Read the model definition and answer for the solid it produces. Units are mm, in the model's axes. Face numbers are marked on the shaded views. Coordinates: 2 decimals unless noted, no trailing zeros. Order: outer loops, then holes, each group sorted by start corner. A loop starts at its lowest first (then second) coordinate and runs counter-clockwise, first axis right, second up. Notation, with made-up numbers: (-15.5, 33) -> (27.5, 33) arc R5 cw to (27.5, 39) -> close; hole circle Ø9 at (33.5, 53.25). An arc over 180 degrees is marked (long way). Answer in a Markdown table with one row per item.
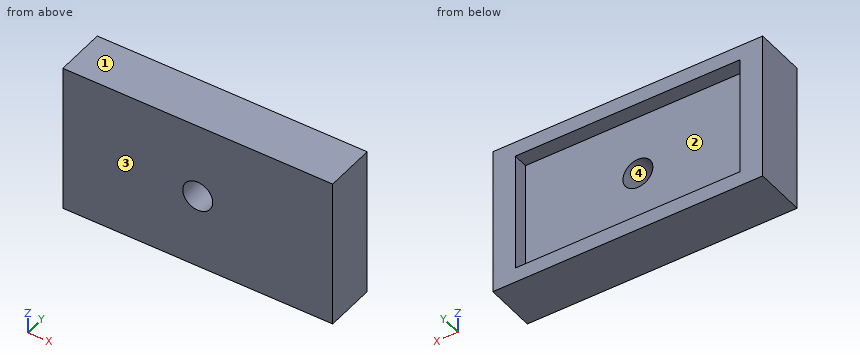
from build123d import *

# Parameters (mm, degrees)
SKETCH1_W           = 90
SKETCH1_H           = 50
BOSS_EXTRUDE1_DEPTH = 17
SKETCH2_W           = 75
SKETCH2_H           = 40
CUT_EXTRUDE1_DEPTH  = 5
SKETCH3_R           = 5
CUT_EXTRUDE2_DEPTH  = 13


with BuildPart() as part:
    # Sketch1 → Boss-Extrude1 (new body)
    with BuildSketch(Plane(origin=(0, 0, 0), x_dir=(1, 0, 0), z_dir=(0, 1, 0))):
        with Locations((45, 25)):
            Rectangle(SKETCH1_W, SKETCH1_H)
    extrude(amount=BOSS_EXTRUDE1_DEPTH)

    # Sketch2 → Cut-Extrude1 (cut)
    with BuildSketch(Plane(origin=(0, 17, 0), x_dir=(1, 0, 0), z_dir=(0, 1, 0))):
        with Locations((45, 25)):
            Rectangle(SKETCH2_W, SKETCH2_H)
    extrude(amount=-CUT_EXTRUDE1_DEPTH, mode=Mode.SUBTRACT)

    # Sketch3 → Cut-Extrude2 (cut, through all)
    with BuildSketch(Plane(origin=(0, 12, 0), x_dir=(1, 0, 0), z_dir=(0, 1, 0))):
        with Locations((45, 25)):
            Circle(SKETCH3_R)
    extrude(amount=-CUT_EXTRUDE2_DEPTH, mode=Mode.SUBTRACT)


solid = part.part
Q1. The part is cut by section C-C (z = -34). Write down the section's boundary in (x, y), then the cut area to 4 significant figures.
Outcome:
| item | result |
|---|---|
| outline | (0, 0) -> (90, 0) -> (90, 17) -> (82.5, 17) -> (82.5, 12) -> (7.5, 12) -> (7.5, 17) -> (0, 17) -> close |
| area | 1,155 mm² |
Q2. The part is cut by section D-D (y = 4.25). Write down the section's boundary in (x, z), then the cut area to 3 significant figures.
Outcome:
| item | result |
|---|---|
| outline | (0, -50) -> (90, -50) -> (90, 0) -> (0, 0) -> close; hole circle Ø10 at (45, -25) |
| area | 4,420 mm² |
Q3. The part is cut by section A-A (x = 45). Write down the section's boundary in (y, z), then the cut area to 3 significant figures.
Outcome:
| item | result |
|---|---|
| outline | (0, -50) -> (17, -50) -> (17, -45) -> (12, -45) -> (12, -30) -> (0, -30) -> close; (0, -20) -> (12, -20) -> (12, -5) -> (17, -5) -> (17, 0) -> (0, 0) -> close |
| area | 530 mm² |
Q4. The part is cut by section B-B (z = -29). Write down the section's boundary in (x, y).
Outcome:
| item | result |
|---|---|
| outline | (0, 0) -> (42, 0) -> (42, 12) -> (7.5, 12) -> (7.5, 17) -> (0, 17) -> close; (48, 0) -> (90, 0) -> (90, 17) -> (82.5, 17) -> (82.5, 12) -> (48, 12) -> close |
Q5. Consider line 1 (X direction, y = 15.75, z = -14); line 2 (Z direction, x = 48, y = 12.75); line 3 (Z direction, x = 45, y = 6.25). Determine where each line is inside the solid, lowest interval first.
Outcome:
| item | result |
|---|---|
| line 1 | 0 to 7.5, 82.5 to 90 |
| line 2 | -50 to -45, -5 to 0 |
| line 3 | -50 to -30, -20 to 0 |
Q6. Given pin 1 (1.5 mm diameter, centred on x = 56.5, z = -21, fed in from +Y), flat-ended and moving along its own axis, determine where the tip first touches the part or whether it passes through.
Outcome:
| item | result |
|---|---|
| pin 1 | y = 12 |
Q7. For a pull along Z with two mould halves and no side action, classify the marked faces 1, 2, 3 and 4 as pulls with the +Z half, pulls with the -Z half, needs draft (parallel to the pull), parting line crosses it, or undercut.
Outcome:
| item | result |
|---|---|
| face 1 | pulls with the +Z half |
| face 2 | undercut |
| face 3 | needs draft |
| face 4 | undercut |
